Input: dimensioned drawing with shaded views. Units: mm. Origin: part minimum x, y, z. Give positions to 0.01 mm unless a question says otherwise; leave off trailing zeros. Write each loop counter-clockwise with the first axis right and the second up, starting at its lowest first coordinate (ties: lowest second). Pieces come first, ordered by that corner, then holes. Notation, with made-up numbers: M 53,70.25 L 82,70.25 A20 cw 82,104.25 Z; hole C -3,67.5 d11. An arc over 180 degrees is marked long. Use CSV: the item, a comma, the result in double quotes. Start each with the question number.
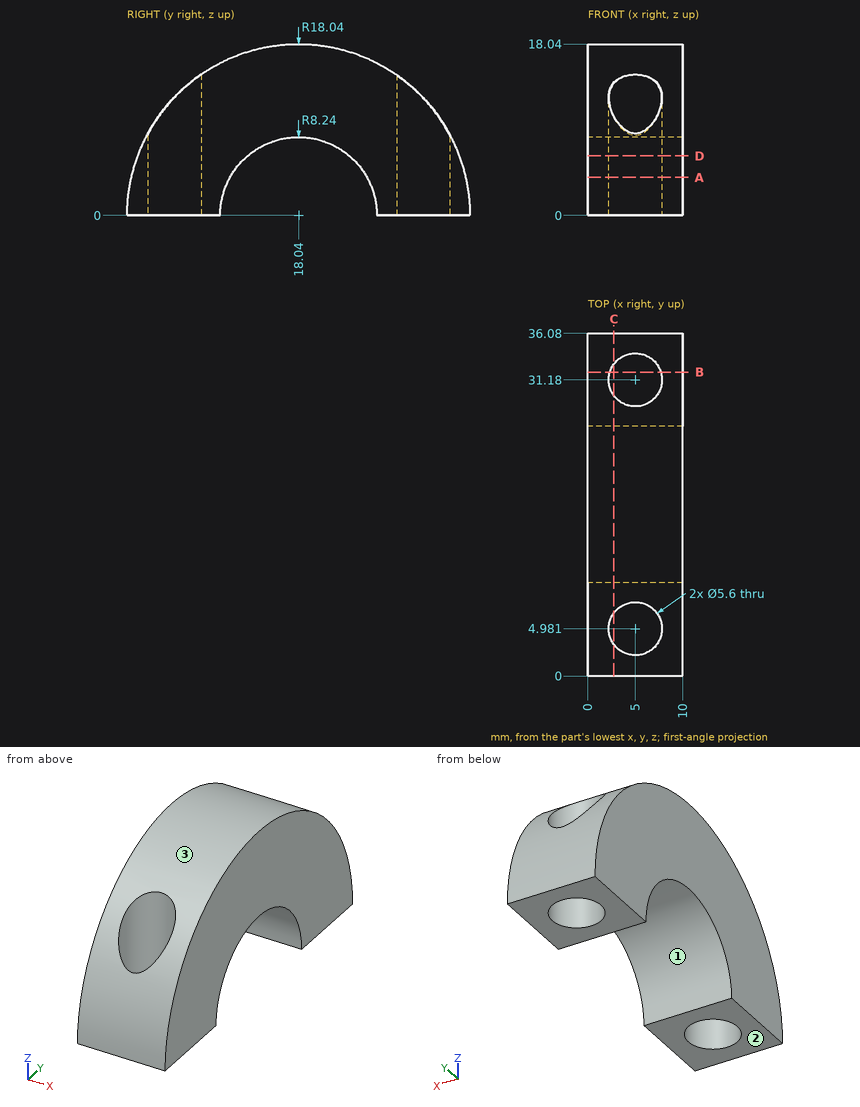
Item 1: Contact query for flat-ended pins moving along their axis: pin 1 Ø1 at (x, y) = (1, 7.5) entering from +Z; pin 2 Ø6 at (x, z) = (2.5, 13) entering from -Y (1 decimal); pin 3 Ø5 at (x, z) = (3, 16) entering from +Y (1 decimal); pin 4 Ø4.5 at (x, y) = (5, 4.98) entering from -Z. Output: stop coordinate, or through.
Item 2: Section C-C (x = 2.75). Return the cut outline in (y, z) (1 decimal).
Item 3: Section B-B (y = 32). Return the cut outline in (x, z), plus the area to 3 significant figures.
Item 4: Material intervals for probe 1 along Y at (x, z) = (5, 7) (1 decimal); probe 2 along Y at (x, z) = (4, 5.5) (1 decimal); probe 3 along Z at (x, y) = (2.75, 18), sorted ascending.
Item 5: Pull-direction query (Y, two-part tool) for the marked faces 1, 2 and 3; classes: released by +Y, released by -Y, zero draft, split by the parting line, or undercut.
Item 6: Section A-A (z = 4). Return the cut outline in (x, y).
Item 7: Section D-D (z = 6.25). Return the cut outline in (x, y).
Output values:
1,pin 1,"stops at z = 14.99"
1,pin 2,"stops at y = 3"
1,pin 3,"stops at y = 29.9"
1,pin 4,"passes through"
2,outline,"M 0,0 L 3.3,0 L 3.3,10.4 A18 ccw Z; M 6.6,0 L 9.8,0 A8.2 cw 26.3,0 L 29.5,0 L 29.5,13.9 A18 ccw 6.6,14 Z; M 32.8,0 L 36.1,0 A18 ccw 32.8,10.3 Z"
3,outline,"M 0,0 L 2.32,0 L 2.32,11.43 L 0,11.43 Z; M 7.68,0 L 10,0 L 10,11.43 L 7.68,11.43 Z"
3,area,"53.1 mm2"
4,probe 1,"y = 1.4 to 2.2, 7.8 to 13.7, 22.4 to 28.4, 34 to 34.7"
4,probe 2,"y = 0.9 to 2.4, 7.6 to 11.9, 24.2 to 28.6, 33.8 to 35.2"
4,probe 3,"z = 8.24 to 18.04"
5,face 1,"undercut"
5,face 2,"zero draft"
5,face 3,"split by the parting line"
6,outline,"M 0,0.45 L 10,0.45 L 10,10.84 L 0,10.84 Z; M 0,25.24 L 10,25.24 L 10,35.63 L 0,35.63 Z; hole C 5,4.98 d5.6; hole C 5,31.18 d5.6"
7,outline,"M 0,1.12 L 10,1.12 L 10,12.67 L 0,12.67 Z; M 0,23.41 L 10,23.41 L 10,34.96 L 0,34.96 Z; hole C 5,4.98 d5.6; hole C 5,31.18 d5.6"
